The model under review builds one solid part; all positions refer to its coordinate system, in mm. A direction names the side the tool comes from. Give positions to 0.01 mm unless a question says otherwise; leave off trailing zeros. Write each loop counter-clockwise with the first axis right and the second up, starting at its lowest first coordinate (ties: lowest second). Pieces come first, ordered by that corner, then holes. Notation, with made-up numbers: (-3.5, 48) - (20.5, 48) arc R24 cw to (20.5, 86) - close; hole circle Ø2 at (46.25, 22). An arc over 180 degrees is marked (long way). Write item = value, one per line.
Autodesk Inventor part; units mm, degrees
ref_plane "YZ Plane" through (0, 0, 0) normal (1, 0, 0) x (0, 1, 0)
ref_plane "XZ Plane" through (0, 0, 0) normal (0, 1, 0) x (-1, 0, 0)
ref_plane "XY Plane" through (0, 0, 0) normal (0, 0, 1) x (1, 0, 0)
sketch "スケッチ1" plane through (0, 0, 0) normal (0, 0, 1) x (1, 0, 0)
  line L0 (20.15, -28.9) -> (-21.15, -28.9)
  line L1 (-21.15, -28.9) -> (-21.15, 22.1)
  line L2 (-21.15, 22.1) -> (20.15, 22.1)
  line L3 (20.15, 22.1) -> (20.15, -28.9)
  line L4 (-16, -1) -> (-16, 1)
  line L5 (16, 1) -> (16, -1)
  line L6 (16, -1) -> (-16, 1) construction
  line L7 (-16, -1) -> (16, 1) construction
  arc A0 (-16, -1) -> (16, -1) centre (0, -1) ccw
  arc A1 (16, 1) -> (-16, 1) centre (0, 1) ccw
  line L8 (-16, 1) -> (-15.8745, 1)
  line L9 (15.8745, 1) -> (16, 1)
  line L10 (16, -1) -> (15.8745, -1)
  line L11 (-15.8745, -1) -> (-16, -1)
  arc A2 (-14.4, 17) -> (-17.6, 17) centre (-16, 17) ccw
  line L12 (-14.4, 17) -> (-14.4, 15)
  line L13 (-17.6, 15) -> (-17.6, 17)
  arc A3 (-17.6, 15) -> (-14.4, 15) centre (-16, 15) ccw
  arc A4 (16.6, 17) -> (13.4, 17) centre (15, 17) ccw
  line L14 (13.4, 15) -> (13.4, 17)
  arc A5 (13.4, 15) -> (16.6, 15) centre (15, 15) ccw
  line L15 (16.6, 17) -> (16.6, 15)
  arc A6 (-14.4, -14) -> (-17.6, -14) centre (-16, -14) ccw
  line L16 (-17.6, -16) -> (-17.6, -14)
  arc A7 (-17.6, -16) -> (-14.4, -16) centre (-16, -16) ccw
  line L17 (-14.4, -14) -> (-14.4, -16)
  arc A8 (16.6, -14) -> (13.4, -14) centre (15, -14) ccw
  line L18 (13.4, -16) -> (13.4, -14)
  arc A9 (13.4, -16) -> (16.6, -16) centre (15, -16) ccw
  line L19 (16.6, -14) -> (16.6, -16)
  point P0 (0, 0)
  point P1 (13.4, -15)
  point P2 (16.6, -15)
  dimension "d5" = 41.3
  dimension "d6" = 51
  dimension "d7" = 2
  dimension "d9" = 16
  dimension "d12" = 2
  dimension "d13" = 1.6
  dimension "d14" = 1.6
  dimension "d17" = 31
  dimension "d20" = 31
  dimension "d29" = 5.15
  dimension "d30" = 14.9
extrude "押し出し1" add sketch "スケッチ1" along normal blind 3
sketch "スケッチ2" plane through (0, 0, 3) normal (0, 0, 1) x (1, 0, 0)
  line L0 (-21.15, -28.9) -> (20.15, -28.9)
  line L1 (-21.15, -28.9) -> (20.15, -28.9)
  line L2 (20.15, -28.9) -> (20.15, -25.9)
  line L3 (20.15, -25.9) -> (-21.15, -25.9)
  line L4 (-21.15, -25.9) -> (-21.15, -28.9)
  point P0 (0, 0)
  dimension "d25" = 3
extrude "押し出し2" add sketch "スケッチ2" along normal blind 33
sketch "スケッチ3" plane through (-21.15, -28.9, 0) normal (0, -1, 0) x (1, 0, 0)
  line L0 (4.75, 19) -> (36.55, 19)
  line L1 (36.55, 19) -> (36.55, 9.5)
  line L2 (36.55, 9.5) -> (4.75, 9.5)
  line L3 (4.75, 9.5) -> (4.75, 19)
  line L4 (0, 0) -> (41.3, 0)
  line L5 (41.3, 0) -> (41.3, 36)
  point P0 (21.15, 0)
  point P1 (36.55, 28.5)
  point P2 (4.75, 28.5)
  dimension "d31" = 9.5
  dimension "d32" = 9.5
  dimension "d33" = 31.8
  dimension "d34" = 4.75
  dimension "d42" = 28.5
hole "穴1" at (-16.4, -28.9, 9.5) at (-16.4, -28.9, 19) at (15.4, -28.9, 9.5) at (15.4, -28.9, 19) at (15.4, -28.9, 28.5) at (-16.4, -28.9, 28.5) direction (0, 1, 0) diameter 4.3 end through all
chamfer "面取り1" distance 3 angle 45 2 edges at (20.15, 22.1, 1.5) (-21.15, 22.1, 1.5)
fillet "フィレット1" radius 3 3 edges at (-21.15, -27.4, 36) (20.15, -27.4, 36) (-0.5, -28.9, 0)
properties part number "ブラケット"
1. Insertion check: P1, Ø5.5, axis at x = -16.4, z = 9.5, coming from the -Y side; P2, Ø20.5, axis at x = 8.5, y = -11.5, coming from the +Z side; P3, Ø5, axis at x = -16.4, z = 19, coming from the +Y side. Each pin has a flat end and moves straight along its axis. Give the tip position at first contact, or say it passes through.
Findings below:
P1 = -28.9
P2 = 3
P3 = -25.9
2. Draft analysis for pull direction X (two halves, no side actions). For faces 1 (the flat face through (-1, -18, 0)), 2 (the flat face through (-21.15, -14, 2)), 3 (the cylindrical face through (-18.21, -27.38, 8.34)), state which applies: +X half, -X half, draft (parallel to the pull), parting line (faces both ways), or undercut.
Findings below:
face_1 = draft
face_2 = -X half
face_3 = undercut
3. Take a section at C-C on y = 0. Give the boundary of the cut face in (x, z).
Findings below:
outline = (-21.15, 0) - (-16, 0) - (-16, 3) - (-21.15, 3) - close; (16, 0) - (20.15, 0) - (20.15, 3) - (16, 3) - close
4. Machinability: for faces 4 (the cylindrical face through (13.27, -27.38, 9.78)), 5 (the cylindrical face through (15, -17.6, 1.5)), which of the approach directions +Z, -Z, +X, -X, +Y, -Y give a long, thin tool a straight path to every point of the face, cutting with its end or side? Answer none if there is none.
Findings below:
face_4 = +Y, -Y
face_5 = +Z, -Z
5. Take a section at A-A on z = 9.5. Give the boundary of the cut face in (x, y).
Findings below:
outline = (-21.15, -28.9) - (-18.55, -28.9) - (-18.55, -25.9) - (-21.15, -25.9) - close; (-14.25, -28.9) - (13.25, -28.9) - (13.25, -25.9) - (-14.25, -25.9) - close; (17.55, -28.9) - (20.15, -28.9) - (20.15, -25.9) - (17.55, -25.9) - close
6. Take a section at B-B on x = 0. Give the boundary of the cut face in (y, z).
Findings below:
outline = (-28.9, 3) arc R3 ccw to (-25.9, 0) - (-17, 0) - (-17, 3) - (-25.9, 3) - (-25.9, 36) - (-28.9, 36) - close; (17, 0) - (22.1, 0) - (22.1, 3) - (17, 3) - close
7. For line 1 (X direction, y = -27, z = 19); line 2 (Z direction, x = 15.4, y = -27.3); line 3 (Z direction, x = -16.4, y = -28), list the stretches that pass through material, from the lowest coordinate up. Write a range as from..to.
Findings below:
line_1 = -21.15..-18.55, -14.25..13.25, 17.55..20.15
line_2 = 0.35..7.35, 11.65..16.85, 21.15..26.35, 30.65..36
line_3 = 0.86..7.35, 11.65..16.85, 21.15..26.35, 30.65..36
8. Take a section at D-D on x = 15.4. Count the separate pieces of the cut face and the enclosed holes in it, and give its area (3 significant figures).
Findings below:
separate_pieces = 7
enclosed_holes = 0
area = 149 mm²
